Read the model definition and answer for the solid it produces. Units are mm, in the model's axes. Face numbers are marked on the shaded views. A direction names the side the tool comes from. Give positions to 0.01 mm unless a question says otherwise; leave off trailing zeros. Write each loop counter-clockwise with the first axis right and the second up, starting at its lowest first coordinate (ties: lowest second). Pieces come first, ordered by that corner, then holes. Notation, with made-up numbers: (49, 33) -> (64, 33) arc R10 cw to (64, 38) -> close; hole circle Ø10 at (-33, 30). An arc over 180 degrees is marked (long way). Put each result on its own line as item: value. Start each with the question number.
Autodesk Inventor part; units mm, degrees
ref_plane "YZ Plane" through (0, 0, 0) normal (1, 0, 0) x (0, 1, 0)
ref_plane "XZ Plane" through (0, 0, 0) normal (0, 1, 0) x (-1, 0, 0)
ref_plane "XY Plane" through (0, 0, 0) normal (0, 0, 1) x (1, 0, 0)
sketch "Sketch2" plane through (0, 0, 0) normal (0, 1, 0) x (-1, 0, 0)
  line L0 (0, 0) -> (-173, 0)
  line L1 (-173, 0) -> (-173, -20)
  line L2 (-173, -20) -> (0, -20)
  line L3 (0, -20) -> (0, 0)
  dimension "d0" = 173
  dimension "d1" = 20
extrude "Extrusion1" add sketch "Sketch2" along normal blind 3
sketch "Sketch3" plane through (0, 3, 0) normal (0, 1, 0) x (1, 0, 0)
  line L0 (173, 20) -> (0, 20)
  line L1 (173, 0) -> (173, 20)
  line L2 (173, 20) -> (173, 0)
  line L3 (15, 20) -> (15, 0)
  line L4 (0, 0) -> (173, 0)
  line L5 (0, 20) -> (0, 0)
  dimension "d8" = 15
bend part "Bend Part1" radius 50 angle 82 line through (15, 3, -20) along (0, 0, 1) centre toward (0, 1, 0) moving side (1, 0, 0) both sides no
properties part number "ball-reload-left"
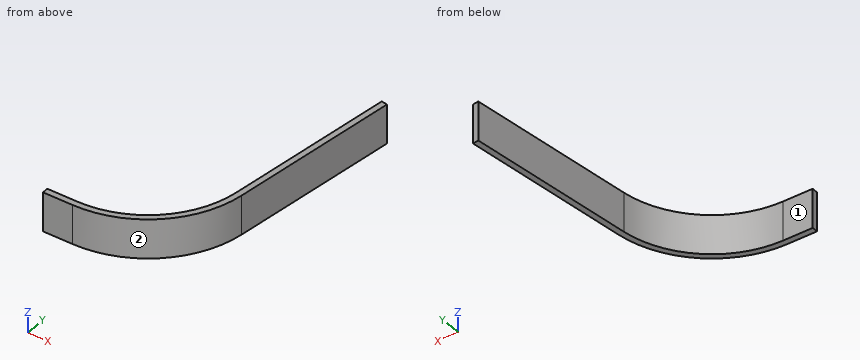
1) A cutting plane is placed at C-C on y = 44. Give the vertices of the cut face in (x, z).
2) A cutting plane is placed at A-A on z = -3.25. Give the vertices of the cut face in (x, y).
3) Each of these flat-tipped pins is pushed along its axis until it touches: pin 1 Ø2 at (y, z) = (28.5, -4) entering from +X; pin 2 Ø2 at (y, z) = (73, -17.5) entering from -X; pin 3 Ø12 at (y, z) = (82, -4) entering from +X. Where does it stop, or does it pass through?
4) Straight lines are drawn through the part: line 1 (Y direction, x = 13.5, z = -7.25); line 2 (Y direction, x = 33, z = -14.75); line 3 (X direction, y = 87, z = -11.5). For each, find the intervals that lie inside material, in ascending order. Write a range as [from, to].
5) A cutting plane is placed at B-B on x = 10. Give the vertices of the cut face in (y, z), and give its area (3 significant figures).
6) For the marked faces 1 and 2, determine the directions among +Z, -Z, +X, -X, +Y, -Y from which every point of the face is accessible in a straight line to the end or side of a thin tool.
Results found:
1. outline: (64.18, -20) -> (67.23, -20) -> (67.23, 0) -> (64.18, 0) -> close
2. outline: (0, 0) -> (15, 0) arc R53 ccw to (67.48, 45.62) -> (79.51, 131.22) -> (76.54, 131.64) -> (64.51, 46.04) arc R50 cw to (15, 3) -> (0, 3) -> close
3. pin 1: stops at x = 62.51
3. pin 2: stops at x = 68.16
3. pin 3: stops at x = 73.44
4. line 1: y = [0, 3]
4. line 2: y = [3.15, 6.35]
4. line 3: x = [70.27, 73.3]
5. outline: (0, -20) -> (3, -20) -> (3, 0) -> (0, 0) -> close
5. area: 60.0 mm²
6. face 1: +Z, -Z, -X, +Y
6. face 2: +Z, -Z, +X, -Y
